from build123d import *
from build123d.topology import SkipClean

# Parameters (mm, degrees)
SKETCH5_W           = 131.802923383
SKETCH5_H           = 32.361272333
CUT_EXTRUDE2_DEPTH  = 27.35
SKETCH7_W           = 25
SKETCH7_H           = 25
BOSS_EXTRUDE1_DEPTH = 40
CUT_EXTRUDE3_START  = -55
SKETCH8_W           = 25
SKETCH8_H           = 25
CUT_EXTRUDE3_DEPTH  = 30
BOSS_EXTRUDE3_START = -40
BOSS_EXTRUDE3_DEPTH = 25
SKETCH10_W          = 6
SKETCH10_H          = 6
CUT_EXTRUDE4_DEPTH  = 25


with BuildPart() as part:
    # Sketch1 → Revolve1 (revolve)
    with BuildSketch(Plane.XY):
        with BuildLine():
            Line((-54.7, 0), (0, 0))
            ThreePointArc((0, 0), (-27.35, 27.35), (-54.7, 0))
        make_face()
        with BuildLine():
            ThreePointArc((0, 0), (27.35, 27.35), (54.7, 0))
            Line((54.7, 0), (0, 0))
        make_face()
    revolve(axis=Axis((0, 0, 0), (1, 0, 0)))

    # Sketch5 → Cut-Extrude2 (cut)
    with SkipClean():  # the faces are left unmerged after this step: merging them gives an invalid solid
        with BuildSketch(Plane(origin=(0, 0, 0), x_dir=(1, 0, 0), z_dir=(0, 1, 0))):
            with Locations((7.898744067, -16.180636167)):
                Rectangle(SKETCH5_W, SKETCH5_H)
        extrude(amount=-CUT_EXTRUDE2_DEPTH, mode=Mode.SUBTRACT)

    # Sketch6 → Revolve2 (revolve)
    with BuildSketch(Plane.XY):
        with BuildLine():
            Line((-42.35, 0), (-12.35, 0))
            ThreePointArc((-12.35, 0), (-27.35, 15), (-42.35, 0))
        make_face()
        with BuildLine():
            ThreePointArc((12.35, 0), (27.35, 15), (42.35, 0))
            Line((42.35, 0), (12.35, 0))
        make_face()
    revolve(axis=Axis((-88.182993462, 0, 0), (1, 0, 0)))

    # Sketch7 → Boss-Extrude1 (add)
    with BuildSketch(Plane.XY):
        with Locations((0, -12.5)):
            Rectangle(SKETCH7_W, SKETCH7_H)
    extrude(amount=-BOSS_EXTRUDE1_DEPTH)

    # Sketch8 → Cut-Extrude3 (cut)
    with BuildSketch(Plane.XY.offset(CUT_EXTRUDE3_START)):
        with Locations((0, -12.5)):
            Rectangle(SKETCH8_W, SKETCH8_H)
        Polygon((9.75, -5.047227516), (-9.75, -5.047227516), (-9.75, -9.747227516), (-4.75, -9.747227516), (-4.75, -15.047227516), (-9.75, -15.047227516), (-9.75, -19.747227516), (9.75, -19.747227516), (9.75, -15.047227516), (4.75, -15.047227516), (4.75, -9.747227516), (9.75, -9.747227516), align=None, mode=Mode.SUBTRACT)
    extrude(amount=CUT_EXTRUDE3_DEPTH, mode=Mode.SUBTRACT)

    # Sketch9 → Boss-Extrude3 (add)
    with BuildSketch(Plane.XY.offset(BOSS_EXTRUDE3_START)):
        Polygon((9.75, -5.047227516), (9.75, -9.747227516), (4.75, -9.747227516), (4.75, -15.047227516), (9.75, -15.047227516), (9.75, -19.747227516), (-9.75, -19.747227516), (-9.75, -15.047227516), (-4.75, -15.047227516), (-4.75, -9.747227516), (-9.75, -9.747227516), (-9.75, -5.047227516), align=None)
    extrude(amount=-BOSS_EXTRUDE3_DEPTH)

    # Sketch10 → Cut-Extrude4 (cut)
    with BuildSketch(Plane.XY):
        with Locations((4, -15.725025673)):
            Rectangle(SKETCH10_W, SKETCH10_H)
        with Locations((-4, -15.725025673)):
            Rectangle(SKETCH10_W, SKETCH10_H)
    extrude(amount=-CUT_EXTRUDE4_DEPTH, mode=Mode.SUBTRACT)


solid = part.part
Verification items for the finished model (mm, model axes). A direction names the side the tool comes from. Coordinates: 2 decimals unless noted, no trailing zeros. Write each loop counter-clockwise with the first axis right and the second up, starting at its lowest first coordinate (ties: lowest second). Pieces come first, ordered by that corner, then holes. Notation, with made-up numbers: M -28.5,43 L -0.5,43 A17 ccw -0.5,71 Z; hole C -4.75,4 d3. An arc over 180 degrees is marked long. Use a Markdown table: item, result.
Q1. Set-up check for faces 1 (the face through (0, -19.747, -45)), 2 (the face through (7, -15.047, -45)), 3 (the face through (-9.75, -17, -45)), 4 (the face through (0, 0, -19)), 5 (the face through (-4, -12.725, -12)): record each of +Z, -Z, +X, -X, +Y, -Y from which the full face is reachable in a straight line by a thin tool's end or side.
Reply:
| item | result |
|---|---|
| face 1 | -Z, +X, -X, -Y |
| face 2 | -Z, +X |
| face 3 | -Z, -X, +Y, -Y |
| face 4 | -Z, +Y |
| face 5 | +Z |
Q2. Sectioned sample at D-D, the plane z = -49.5. Record the boundary of the cut face in (x, y), plus the area to 3 significant figures.
Reply:
| item | result |
|---|---|
| outline | M -9.75,-19.75 L 9.75,-19.75 L 9.75,-15.05 L 4.75,-15.05 L 4.75,-9.75 L 9.75,-9.75 L 9.75,-5.05 L -9.75,-5.05 L -9.75,-9.75 L -4.75,-9.75 L -4.75,-15.05 L -9.75,-15.05 Z |
| area | 234 mm² |
Q3. Go/stop test with flat-tipped pins: P1, Ø4, axis at x = 7.5, z = -43.5, coming from the +Y side; P2, Ø8, axis at x = -8.5, z = -16, coming from the -Y side; P3, Ø4, axis at x = 6.5, z = -54, coming from the -Y side. Record where each tip stops, or that it passes through.
Reply:
| item | result |
|---|---|
| P1 | stops at y = -5.05 |
| P2 | stops at y = -25 |
| P3 | stops at y = -19.75 |
Q4. Sectioned sample at A-A, the plane z = 2. Record the boundary of the cut face in (x, y), plus the area to 3 significant figures.
Reply:
| item | result |
|---|---|
| outline | M -54.63,0 L -42.22,0 A14.87 ccw -12.48,0 L -0.07,0 A27.28 ccw Z; M 0.07,0 L 12.48,0 A14.87 ccw 42.22,0 L 54.63,0 A27.28 ccw Z |
| area | 3,030 mm² |
Q5. Thickness scan on line 1 (X direction, y = -3, z = 11); line 2 (Z direction, x = -11.5, y = -17); line 3 (Y direction, x = -3, z = -43.5). Record the ranges inside material, lowest first.
Reply:
| item | result |
|---|---|
| line 1 | x = -37.1 to -17.6, 17.6 to 37.1 |
| line 2 | z = -25 to 0 |
| line 3 | y = -19.75 to -5.05 |
Q6. Draft check along Y on faces 6 (the face through (-9.75, -7, -45)), 7 (the face through (1, -16, -12)), 8 (the face through (0, -25, -12)), 9 (the face through (-3, -16, -25)). Enter one of: +Y half, -Y half, draft (parallel to the pull), parting line (faces both ways), or undercut.
Reply:
| item | result |
|---|---|
| face 6 | draft |
| face 7 | undercut |
| face 8 | -Y half |
| face 9 | undercut |
Q7. Sectioned sample at C-C, the plane y = -8. Record the boundary of the cut face in (x, z).
Reply:
| item | result |
|---|---|
| outline | M -53.5,0 A26.15 ccw -12.5,-21.53 L -12.5,-25 L -9.75,-25 L -9.75,-65 L 9.75,-65 L 9.75,-25 L 12.5,-25 L 12.5,-21.53 A26.15 ccw 53.5,0 L 40.04,0 A12.69 ccw 14.66,0 L -14.66,0 A12.69 ccw -40.04,0 Z |
Q8. Sectioned sample at B-B, the plane z = -12. Record the boundary of the cut face in (x, y), plus the area to 3 significant figures.
Reply:
| item | result |
|---|---|
| outline | M -12.5,-25 L 12.5,-25 L 12.5,-19.58 A24.58 ccw long 2.77,0 L -2.77,0 A24.58 ccw long -12.5,-19.58 Z; hole M -7,-18.73 L -1,-18.73 L -1,-12.73 L -7,-12.73 Z; hole M 1,-18.73 L 7,-18.73 L 7,-12.73 L 1,-12.73 Z |
| area | 4,080 mm² |
